Check sheet for the modelled part. Datum: model origin and axes. Units: mm. A direction names the side the tool comes from. Give positions to 0.01 mm unless a question says otherwise; leave off trailing zeros. Order: outer loops, then holes, each group sorted by start corner. A loop starts at its lowest first (then second) coordinate and runs counter-clockwise, first axis right, second up.
Item 1: Sectioned sample at D-D on x = 17.25. Record the boundary of the cut face in (y, z), and give its area (3 significant figures).
Item 2: Material ranges on line 1 along X through (y, z) = (-5.25, -7.75); line 2 along X through (y, z) = (-3.25, -2); line 3 along Z through (x, y) = (10.75, 1), recorded low to high.
Item 3: Sectioned sample at A-A on y = 0. Record the boundary of the cut face in (x, z).
Item 4: Gauge pin test, flat ends, axial feed: P1, Ø1, axis at x = 7, z = -5.5, coming from the +Y side; P2, Ø10, axis at x = 17.5, y = -4.5, coming from the +Z side; P3, Ø8, axis at x = 11.5, z = -1, coming from the -Y side; P4, Ø5, axis at y = -5.5, z = 4, coming from the -X side. Record the tip position at first contact, or that the pin passes through.
Item 5: Access from +Z, -Z, +X, -X, +Y, -Y to the whole of each face (thin tool, end or side, straight path). Record for faces 1 (the cylindrical face through (14.86, -0.867, -3.905)), 2 (the flat face through (0, 0, 0)).
Item 6: Sectioned sample at C-C on x = 3.25. Record the boundary of the cut face in (y, z).
from build123d import *

# Parameters (mm, degrees)
F2_SIZE = 0.5


with BuildPart() as f1:
    # F0 (on Top) → F1 (revolve)
    with BuildSketch(Plane.XY):
        Polygon((0, 3), (0, 0), (28, 0), (28, 10), (25, 10), (25, 4), (5, 4), (5, 3), align=None)
    revolve(axis=Axis((27.980929, 0, 0), (1, 0, 0)))

    # F2
    f2_edges = [f1.edges().sort_by_distance(p)[0] for p in [
        (28, -10, 0),
        (25, -10, 0),
    ]]
    chamfer(f2_edges, length=F2_SIZE)


solid = f1.part
Report:
1. outline: circle Ø8 at (0, 0)
1. area: 50.3 mm2
2. line 1: x = 25 to 28
2. line 2: x = 5 to 28
2. line 3: z = -3.87 to 3.87
3. outline: (0, -3) - (5, -3) - (5, -4) - (25, -4) - (25, -9.5) - (25.5, -10) - (27.5, -10) - (28, -9.5) - (28, 9.5) - (27.5, 10) - (25.5, 10) - (25, 9.5) - (25, 4) - (5, 4) - (5, 3) - (0, 3) - close
4. P1: passes through
4. P2: stops at z = 4
4. P3: stops at y = -4
4. P4: stops at x = 25
5. face 1: -X
5. face 2: +Z, -Z, -X, +Y, -Y
6. outline: circle Ø6 at (0, 0)
